For this review, take the finished solid that the model builds, in its own axes (mm). Face numbers are marked on the shaded views. A direction names the side the tool comes from. Round coordinates to 2 decimals unless told otherwise and drop trailing zeros. Loops run counter-clockwise (first coordinate to the right, second up) from the corner with the lowest first, then second, coordinate; pieces in that order, holes last. Notation, with made-up numbers: (-15.5, 67) -> (34.5, 67) arc R12 cw to (34.5, 88) -> close; hole circle Ø10 at (5.5, -11.75). An arc over 180 degrees is marked (long way). Write each question's results on one line, items separated by ' | '.
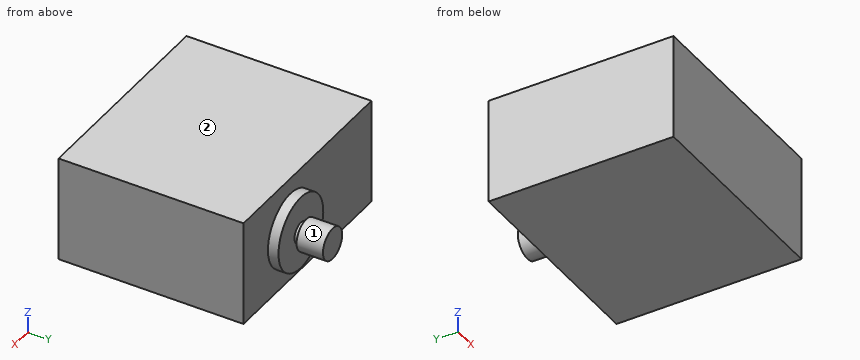
```python
from build123d import *

# Parameters (mm, degrees)
SKETCH_1_W      = 40
SKETCH_1_H      = 35
EXTRUDE_1_DEPTH = 10


with BuildPart() as part:
    # ｽｹｯﾁ1 → ﾎﾞｽ - 押し出し1 (new, symmetric)
    with BuildSketch(Plane.XY):
        with Locations((20, 17.5)):
            Rectangle(SKETCH_1_W, SKETCH_1_H)
    extrude(amount=EXTRUDE_1_DEPTH, both=True)

    # ｽｹｯﾁ2 → 回転1 (revolve)
    with BuildSketch(Plane.XY, mode=Mode.PRIVATE) as revolve_1_sk:
        Polygon((25.364248034, 35), (25.364248034, 43), (22.364248034, 43), (22.364248034, 38), (23.364248034, 38), (23.364248034, 37), (18.364248034, 37), (18.364248034, 35), align=None)
    revolve(revolve_1_sk.sketch.rotate(Axis((25.364248034, 35, 0), (0, 1, 0)), 270), axis=Axis((25.364248034, 35, 0), (0, 1, 0)))


solid = part.part
```
1. For pin 1 (3 mm diameter, centred on x = 20, z = 1.5, fed in from +Y); pin 2 (6 mm diameter, centred on x = 11, z = 7, fed in from +Y), all flat-tipped, find the tip position at first contact; note any pin that passes through.
Values found:
pin 1: stops at y = 37 | pin 2: stops at y = 35
2. Consider section B-B (z = 2.5). State the section outline as (x, y) points, plus the area to 3 significant figures.
Values found:
outline: (0, 0) -> (40, 0) -> (40, 35) -> (31.9, 35) -> (31.9, 37) -> (18.83, 37) -> (18.83, 35) -> (0, 35) -> close; (23.71, 38) -> (27.02, 38) -> (27.02, 43) -> (23.71, 43) -> close | area: 1,440 mm2
3. To check wall thickness, follow probe 1 along Y at (x, z) = (13, -7.5); probe 2 along X at (y, z) = (36, 0.25); probe 3 along Y at (x, z) = (30, -0.5). State the ranges of each line that lie inside material, in increasing order.
Values found:
probe 1: y = 0 to 35 | probe 2: x = 18.37 to 32.36 | probe 3: y = 0 to 37
4. Consider section D-D (z = 7.5). State the section outline as (x, y) points.
Values found:
outline: (0, 0) -> (40, 0) -> (40, 35) -> (0, 35) -> close
5. Consider section C-C (x = 19). State the section outline as (y, z) points.
Values found:
outline: (0, -10) -> (35, -10) -> (35, -2.91) -> (37, -2.91) -> (37, 2.91) -> (35, 2.91) -> (35, 10) -> (0, 10) -> close
6. Tool access review of the marked faces 1 and 2: name each direction out of +Z, -Z, +X, -X, +Y, -Y from which nothing blocks a thin tool from reaching the whole face with its end or side.
Values found:
face 1: +Y | face 2: +Z, +X, -X, +Y, -Y
7. Consider section A-A (z = 0). State the section outline as (x, y) points, plus the area to 3 significant figures.
Values found:
outline: (0, 0) -> (40, 0) -> (40, 35) -> (32.36, 35) -> (32.36, 37) -> (27.36, 37) -> (27.36, 38) -> (28.36, 38) -> (28.36, 43) -> (22.36, 43) -> (22.36, 38) -> (23.36, 38) -> (23.36, 37) -> (18.36, 37) -> (18.36, 35) -> (0, 35) -> close | area: 1,460 mm2
